from build123d import *

# Parameters (mm, degrees)
EXTRUDE002_DEPTH  = 4
TUBE029_R         = 57.75
TUBE029_R_2       = 55.25
TUBE029_DEPTH     = 15
TUBE027_R         = 51.9
TUBE027_R_2       = 49.4
TUBE027_DEPTH     = 15
TUBE030_R         = 10.9
TUBE030_R_2       = 8.9
TUBE030_DEPTH     = 11
TUBE031_R         = 8.9
TUBE031_R_2       = 4.1
TUBE031_DEPTH     = 2.5
ARRAY034_COUNT    = 3
CYLINDER030_R     = 8.9
CYLINDER030_DEPTH = 4
ARRAY033_COUNT    = 3
CYLINDER029_R     = 49.4
CYLINDER029_DEPTH = 4
TUBE028_R         = 55.25
TUBE028_R_2       = 51.75
TUBE028_DEPTH     = 5


with BuildPart() as valvecutter:
    # Face002 → Extrude002 (new body)
    with BuildSketch(Plane(origin=(0, 0, 0), x_dir=(0, 1, 0), z_dir=(0, 0, 1))):
        Polygon((0, -4.2), (3.637307, -2.1), (3.637307, 2.1), (0, 4.2), (-3.637307, 2.1), (-3.637307, -2.1), align=None)
    extrude(amount=EXTRUDE002_DEPTH)


with BuildPart() as valvecutter_1:
    # Extrude002 placement: moved
    add(valvecutter.part.moved(Location((30, 0, -5))))


with BuildPart() as lidconnectorouter:
    # Tube029 → Tube029 (new body)
    with BuildSketch(Plane.XY.offset(-5)):
        Circle(TUBE029_R)
        Circle(TUBE029_R_2, mode=Mode.SUBTRACT)
    extrude(amount=TUBE029_DEPTH)


with BuildPart() as lidconnectorinner:
    # Tube027 → Tube027 (new body)
    with BuildSketch(Plane.XY.offset(-5)):
        Circle(TUBE027_R)
        Circle(TUBE027_R_2, mode=Mode.SUBTRACT)
    extrude(amount=TUBE027_DEPTH)


with BuildPart() as lidrailguide:
    # Tube030 → Tube030 (new body)
    with BuildSketch(Plane(origin=(-40.5, 0, -1), x_dir=(1, 0, 0), z_dir=(0, 0, 1))):
        Circle(TUBE030_R)
        Circle(TUBE030_R_2, mode=Mode.SUBTRACT)
    extrude(amount=TUBE030_DEPTH)


with BuildPart() as lidrailguides:
    # Tube031 → Tube031 (new body)
    with BuildSketch(Plane(origin=(-40.5, 0, 7.5), x_dir=(1, 0, 0), z_dir=(0, 0, 1))):
        Circle(TUBE031_R)
        Circle(TUBE031_R_2, mode=Mode.SUBTRACT)
    extrude(amount=TUBE031_DEPTH)

    # Fusion016: union LidRailGuide
    add(lidrailguide.part)

    # Array034: LidRailGuides ×3 about axis
    array034_axis = Axis((0, 0, 0), (0, 0, 1))


with BuildPart() as lidrailguides_1:
    add(lidrailguides.part)
    for i in range(1, ARRAY034_COUNT):
        add(lidrailguides.part.rotate(array034_axis, i * 360 / ARRAY034_COUNT))


with BuildPart() as lidnutcutters:
    # Cylinder030 → Cylinder030 (new body)
    with BuildSketch(Plane(origin=(-40.5, 0, -5), x_dir=(1, 0, 0), z_dir=(0, 0, 1))):
        Circle(CYLINDER030_R)
    extrude(amount=CYLINDER030_DEPTH)

    # Array033: LidNutCutters ×3 about axis
    array033_axis = Axis((0, 0, 0), (0, 0, 1))


with BuildPart() as lidnutcutters_1:
    add(lidnutcutters.part)
    for i in range(1, ARRAY033_COUNT):
        add(lidnutcutters.part.rotate(array033_axis, i * 360 / ARRAY033_COUNT))


with BuildPart() as lid1:
    # Cylinder029 → Cylinder029 (new body)
    with BuildSketch(Plane.XY.offset(-5)):
        Circle(CYLINDER029_R)
    extrude(amount=CYLINDER029_DEPTH)

    # Cut056: cut LidNutCutters
    add(lidnutcutters_1.part, mode=Mode.SUBTRACT)


with BuildPart() as lid3:
    # Tube028 → Tube028 (new body)
    with BuildSketch(Plane.XY.offset(-5)):
        Circle(TUBE028_R)
        Circle(TUBE028_R_2, mode=Mode.SUBTRACT)
    extrude(amount=TUBE028_DEPTH)

    # Fusion017: union LidConnectorOuter, LidConnectorInner, LidRailGuides, Lid1
    add(lidconnectorouter.part)
    add(lidconnectorinner.part)
    add(lidrailguides_1.part)
    add(lid1.part)

    # Cut057: cut ValveCutter
    add(valvecutter_1.part, mode=Mode.SUBTRACT)


solid = lid3.part
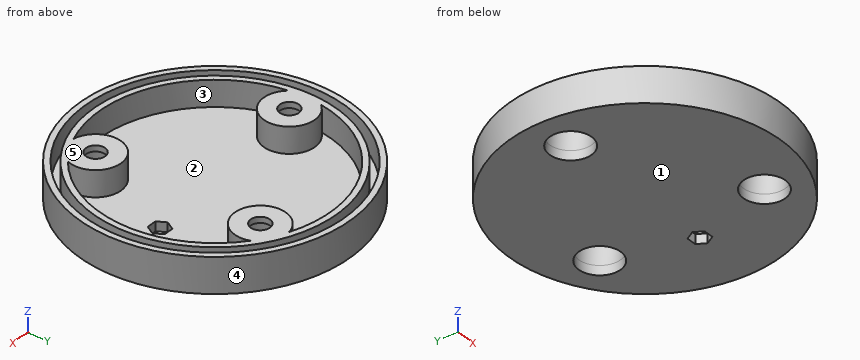
Read the model definition and answer for the solid it produces. Units are mm, in the model's axes. Face numbers are marked on the shaded views. A direction names the side the tool comes from. Give positions to 0.01 mm unless a question says otherwise; leave off trailing zeros. Write each loop counter-clockwise with the first axis right and the second up, starting at its lowest first coordinate (ties: lowest second). Pieces come first, ordered by that corner, then holes. Notation, with made-up numbers: (-30, 24.5) - (29, 24.5) arc R19 cw to (29, 45.5) - close; hole circle Ø8 at (7, 4.5). An arc over 180 degrees is marked (long way). Use CSV: the item, a comma, the result in double quotes. Start each with the question number.
Item 1: Consider line 1 (Y direction, x = 0, z = 4.75); line 2 (Y direction, x = -28.5, z = 5.25); line 3 (X direction, y = -42, z = 3.5). Determine where each line is inside the solid, lowest interval first.
Item 2: Flat-ended cylindrical pins translate along their axes: P1, Ø6, axis at y = 37.5, z = 4.5, coming from the -X side; P2, Ø5, axis at y = 16.5, z = 1, coming from the +X side; P3, Ø8, axis at x = 22.5, z = 7, coming from the -Y side. Find the tip coordinate at first contact, or state that the pin passes through.
Item 3: The part is cut by section A-A, the plane z = 2.75. Give the vertices of the cut face in (x, y), and give its area (3 significant figures).
Item 4: The part is cut by section D-D, the plane x = 0. Give the vertices of the cut face in (y, z), and give its area (3 significant figures).
Item 5: The mould has two halves that part along X. Classify the marked faces 3, 4 and 5: pulls with the +X half, pulls with the -X half, needs draft (parallel to the pull), parting line crosses it, or undercut.
Item 6: The part is cut by section C-C, the plane y = 2. Give the vertices of the cut face in (x, z).
Item 7: The part is cut by section B-B, the plane x = -40.5. Give the vertices of the cut face in (y, z), and give its area (3 significant figures).
Item 8: For the marked faces 1 and 2, determine the directions among +Z, -Z, +X, -X, +Y, -Y from which every point of the face is accessible in a straight line to the end or side of a thin tool.
Taken from the geometry:
1,line 1,"-57.75 to -55.25, -51.9 to -49.4, 49.4 to 51.9, 55.25 to 57.75"
1,line 2,"-50.23 to -47.33, -43.37 to -40.35, 40.35 to 43.37, 47.33 to 50.23"
1,line 3,"-39.64 to -35.9, -30.49 to -26.01, 11.83 to 14.66, 25.84 to 30.49, 35.9 to 39.64"
2,P1,"x = -46.31"
2,P2,"x = 56.03"
2,P3,"y = -54.71"
3,outline,"circle Ø115.5 at (0, 0); circle Ø103.8 at (0, 0); hole circle Ø110.5 at (0, 0); hole circle Ø17.8 at (-40.5, 0); hole (-48.91, -6.93) arc R49.4 ccw to (18.45, -45.82) arc R10.9 cw (long way) to (30.46, -38.89) arc R49.4 ccw to (30.46, 38.89) arc R10.9 cw (long way) to (18.45, 45.82) arc R49.4 ccw to (-48.91, 6.93) arc R10.9 cw (long way) to start; hole circle Ø17.8 at (20.25, -35.07); hole circle Ø17.8 at (20.25, 35.07)"
3,area,"2,000 mm2"
4,outline,"(-57.75, -5) - (57.75, -5) - (57.75, 10) - (55.25, 10) - (55.25, 0) - (51.9, 0) - (51.9, 10) - (49.4, 10) - (49.4, -1) - (-49.4, -1) - (-49.4, 10) - (-51.9, 10) - (-51.9, 0) - (-55.25, 0) - (-55.25, 10) - (-57.75, 10) - close"
4,area,"579 mm2"
5,face 3,"undercut"
5,face 4,"parting line crosses it"
5,face 5,"needs draft"
6,outline,"(-57.72, -5) - (-49.17, -5) - (-49.17, 7.5) - (-44.08, 7.5) - (-44.08, 10) - (-51.86, 10) - (-51.86, 0) - (-55.21, 0) - (-55.21, 10) - (-57.72, 10) - close; (-36.92, 7.5) - (-31.83, 7.5) - (-31.83, -5) - (26.95, -5) - (26.95, -1) - (-29.79, -1) - (-29.79, 10) - (-36.92, 10) - close; (33.05, -5) - (57.72, -5) - (57.72, 10) - (55.21, 10) - (55.21, 0) - (51.86, 0) - (51.86, 10) - (49.36, 10) - (49.36, -1) - (33.05, -1) - close"
7,outline,"(-41.17, -5) - (-8.9, -5) - (-8.9, 7.5) - (-4.1, 7.5) - (-4.1, 10) - (-10.9, 10) - (-10.9, -1) - (-28.29, -1) - (-28.29, 10) - (-32.46, 10) - (-32.46, 0) - (-37.58, 0) - (-37.58, 10) - (-41.17, 10) - close; (4.1, 7.5) - (8.9, 7.5) - (8.9, -5) - (41.17, -5) - (41.17, 10) - (37.58, 10) - (37.58, 0) - (32.46, 0) - (32.46, 10) - (28.29, 10) - (28.29, -1) - (10.9, -1) - (10.9, 10) - (4.1, 10) - close"
7,area,"507 mm2"
8,face 1,"-Z, +X, -X, +Y, -Y"
8,face 2,"+Z"
